Part model, mm, in its own coordinate system. Give positions to 0.01 mm unless a question says otherwise; leave off trailing zeros. Write each loop counter-clockwise with the first axis right and the second up, starting at its lowest first coordinate (ties: lowest second). Pieces come first, ordered by that corner, then holes.
from build123d import *

# Parameters (mm, degrees)
MAIN_PLATE_SIZE_DEPTH                         = 6.35
SKETCH2_R                                     = 9.525
SKETCH2_R_2                                   = 1.778
BOTTOM_SHAFT_MOUNTING_HOLES_DEPTH             = 486.307863629
SKETCH3_R                                     = 6.35
SKETCH3_R_2                                   = 1.778
TOP_BATTERY_BOX_MOUNTING_HOLES_DEPTH          = 486.307863629
THIS_IS_TO_MATCH_THE_IDIOTIC_DESIGN_OF_B_SIZE = 6.35
THIS_IS_TO_MATCH_THE_IDIOTIC_DESIGN_2_R       = 10
SKETCH4_R                                     = 2.5
F_20MM_EXTRUSION_MOUNT_DEPTH                  = 486.307863629


with BuildPart() as part:
    # Sketch1 → Main Plate Size (new body)
    with BuildSketch(Plane(origin=(0, 0, 0), x_dir=(0, 0, -1), z_dir=(1, 0, 0))):
        Polygon((330.2, 112.361360549), (86.961360549, 355.6), (0, 355.6), (0, 0), (330.2, 0), align=None)
    extrude(amount=MAIN_PLATE_SIZE_DEPTH)

    # Sketch2 → Bottom Shaft Mounting Holes (cut, through all)
    with BuildSketch(Plane(origin=(6.35, 0, 0), x_dir=(0, 0, -1), z_dir=(1, 0, 0))):
        with BuildLine():
            Line((134.1120127, 20.8026), (0, 20.8026))
            Line((0, 20.8026), (0, 0))
            Line((0, 0), (159.512000023, 0))
            ThreePointArc((159.512000023, 0), (143.096249024, 5.864358018), (134.1120127, 20.8026))
        make_face()
        with BuildLine():
            ThreePointArc((184.9119873, 20.8026), (175.927750994, 5.864358033), (159.512000023, 0))
            Line((159.512000023, 0), (177.8, 0))
            Line((177.8, 0), (330.2, 0))
            Line((330.2, 0), (330.2, 20.8026))
            Line((330.2, 20.8026), (184.9119873, 20.8026))
        make_face()
        with Locations((159.512, 23.8252)):
            Circle(SKETCH2_R)
        with Locations((159.512, 4.7752)):
            Circle(SKETCH2_R_2)
        with Locations((178.562, 23.8252)):
            Circle(SKETCH2_R_2)
        with Locations((159.512, 42.8752)):
            Circle(SKETCH2_R_2)
        with Locations((140.462, 23.8252)):
            Circle(SKETCH2_R_2)
    extrude(amount=-BOTTOM_SHAFT_MOUNTING_HOLES_DEPTH, mode=Mode.SUBTRACT)

    # Sketch3 → Top Battery Box Mounting Holes (cut, through all)
    with BuildSketch(Plane(origin=(6.35, 0, 0), x_dir=(0, 0, -1), z_dir=(1, 0, 0))):
        with Locations((159.512, 106.5022)):
            Circle(SKETCH3_R)
        with Locations((149.733, 106.5022)):
            Circle(SKETCH3_R_2)
        with Locations((159.512, 116.2812)):
            Circle(SKETCH3_R_2)
        with Locations((169.291, 106.5022)):
            Circle(SKETCH3_R_2)
        with Locations((159.512, 96.7232)):
            Circle(SKETCH3_R_2)
    extrude(amount=-TOP_BATTERY_BOX_MOUNTING_HOLES_DEPTH, mode=Mode.SUBTRACT)

    # This is to match the idiotic Design of B
    # the kernel refuses this chamfer: 6.35 mm, written as the material it adds along each edge
    with BuildSketch(Plane(origin=(6.35, 20.8026, -134.1120127), x_dir=(0, -0.9387383646661523, -0.34463064678568256), z_dir=(-1, 0, 0))) as this_is_to_match_the_idiotic_design_of_b_piece_1:
        with BuildLine():
            Line((7.921958409, 0), (-THIS_IS_TO_MATCH_THE_IDIOTIC_DESIGN_OF_B_SIZE * 0.344630646786, THIS_IS_TO_MATCH_THE_IDIOTIC_DESIGN_OF_B_SIZE * 0.938738364666))
            Line((-THIS_IS_TO_MATCH_THE_IDIOTIC_DESIGN_OF_B_SIZE * 0.344630646786, THIS_IS_TO_MATCH_THE_IDIOTIC_DESIGN_OF_B_SIZE * 0.938738364666), (0, 0))
            ThreePointArc((0, 0), (4.071959946, 0.304342453), (7.921958409, 0))
        make_face()
    extrude(amount=6.35)
    with BuildSketch(Plane(origin=(6.35, 20.8026, -184.9119873), x_dir=(0, 0, -1), z_dir=(-1, 0, 0))) as this_is_to_match_the_idiotic_design_of_b_piece_2:
        with BuildLine():
            Line((THIS_IS_TO_MATCH_THE_IDIOTIC_DESIGN_OF_B_SIZE, 0), (-2.73014965, 7.436646282))
            ThreePointArc((-2.73014965, 7.436646282), (-1.117624253, 3.927390757), (0, 0))
            Line((0, 0), (THIS_IS_TO_MATCH_THE_IDIOTIC_DESIGN_OF_B_SIZE, 0))
        make_face()
    extrude(amount=6.35)

    # This is to match the idiotic Design  2
    this_is_to_match_the_idiotic_design_2_edges = [part.edges().sort_by_distance(p)[0] for p in [
        (3.175, 13.365953718, -136.84216235),
        (3.175, 13.365953718, -182.18183765),
        (3.175, 20.8026, -191.2619873),
        (3.175, 20.8026, -127.7620127),
    ]]
    fillet(this_is_to_match_the_idiotic_design_2_edges, radius=THIS_IS_TO_MATCH_THE_IDIOTIC_DESIGN_2_R)

    # Sketch4 → 20mm Extrusion Mount (cut, through all)
    with BuildSketch(Plane(origin=(6.35, 0, 0), x_dir=(0, 0, -1), z_dir=(1, 0, 0))):
        with Locations((10, 97.0026)):
            Circle(SKETCH4_R)
    extrude(amount=-F_20MM_EXTRUSION_MOUNT_DEPTH, mode=Mode.SUBTRACT)


solid = part.part
1) Drill centre lines: L1, parallel to Z at x = 5, y = 96.5; L2, parallel to Y at x = 2.5, z = -155; L3, parallel to Y at x = 2.5, z = -40.5. Where is each one in solid material? Low to high.
Check result:
L1: z = -330.2 to -161.28, -157.75 to -12.45, -7.55 to 0
L2: y = 0.4 to 15.44, 32.21 to 102.03, 110.97 to 287.56
L3: y = 20.8 to 355.6
2) Saw through at B-B (z = -71.5). Write the cut outline in (x, y).
Check result:
outline: (0, 20.8) - (6.35, 20.8) - (6.35, 355.6) - (0, 355.6) - close
3) Mould opens along Y. For faces 1 (the cylindrical face through (3.2, 102.6, -154.5)), 2 (the cylindrical face through (3.22, 20.18, -168.31)), 3 (the flat face through (3.13, 232.28, -210.28)), 4 (the flat face through (0, 175, -126)) say: +Y half, -Y half, draft (parallel to the pull), parting line (faces both ways), or undercut.
Check result:
face 1: undercut
face 2: undercut
face 3: +Y half
face 4: draft
4) Saw through at C-C (y = 172). Write the cut outline in (x, z).
Check result:
outline: (0, -270.56) - (6.35, -270.56) - (6.35, 0) - (0, 0) - close
5) Saw through at A-A (x = 2). State how many separate pieces and enclosed holes the cut face has, and give its area (3 significant figures).
Check result:
separate pieces: 1
enclosed holes: 11
area: 81,300 mm2
6) Flat gauge pins, fed straight in: P1, Ø2, axis at x = 3.5, y = 122, coming from the -Z side; P2, Ø3, axis at y = 96.72, z = -159.51, coming from the +X side; P3, Ø1.9, axis at x = 4.5, z = -57, coming from the -Y side; P4, Ø5.5, axis at y = 42.88, z = -159.51, coming from the -X side. Where does each tip first touch, or does it go through?
Check result:
P1: stops at z = -321.56
P2: passes through
P3: stops at y = 20.8
P4: stops at x = 0
